Model file for the job. Use its own axes, mm. A direction names the side the tool comes from. Coordinates: 2 decimals unless noted, no trailing zeros. Write each loop counter-clockwise with the first axis right and the second up, starting at its lowest first coordinate (ties: lowest second). Pieces come first, ordered by that corner, then holes. Notation, with made-up numbers: (8.5, 65.5) -> (22.5, 65.5) arc R14 cw to (22.5, 71.5) -> close; hole circle Ø6 at (62.5, -16.5). An arc over 180 degrees is marked (long way). Answer as a JSON object with one key per item and string values. Group by question number.
from build123d import *

# Parameters (mm, degrees)
SKETCH1_W                = 37
SKETCH1_H                = 28
SKETCH1_R                = 1.75
BOSS_EXTRUDE1_DEPTH      = 7.8
BOSS_EXTRUDE2_DEPTH      = 10
BOSS_EXTRUDE2_DEPTH_BACK = 2
SKETCH1_3_W              = 44
SKETCH1_3_H              = 35
SKETCH1_3_W_2            = 37
SKETCH1_3_H_2            = 28
SKETCH1_3_W_3            = 8
SKETCH1_3_H_3            = 3
FILLET1_R                = 9
CUT_EXTRUDE1_DEPTH       = 2.1
HOLE1_D                  = 3.3


with BuildPart() as part:
    # Sketch1 → Boss-Extrude1 (new body)
    with BuildSketch(Plane.XY):
        Polygon((-7.2, 0), (0, 0), (0, 32), (8, 32), (8, 35), (-52, 35), (-52, 32), (-44, 32), (-44, 0), (-36.8, 0), (-36.8, -12), (-7.2, -12), align=None)
        with Locations((-22, 17.5)):
            Rectangle(SKETCH1_W, SKETCH1_H, mode=Mode.SUBTRACT)
        with Locations((-15, -8.4)):
            Circle(SKETCH1_R, mode=Mode.SUBTRACT)
        with Locations((-29, -8.4)):
            Circle(SKETCH1_R, mode=Mode.SUBTRACT)
    extrude(amount=BOSS_EXTRUDE1_DEPTH)

    # Sketch1<3> → Boss-Extrude2 (add, two sides: drawn at the far end of the back side and taken through both)
    # profile 1 of 3: a face of its own
    with BuildSketch(Plane.XY.offset(-BOSS_EXTRUDE2_DEPTH_BACK)):
        with Locations((-22, 17.5)):
            Rectangle(SKETCH1_3_W, SKETCH1_3_H)
        with Locations((-22, 17.5)):
            Rectangle(SKETCH1_3_W_2, SKETCH1_3_H_2, mode=Mode.SUBTRACT)
    # profile 2 of 3: a face of its own
    with BuildSketch(Plane.XY.offset(-BOSS_EXTRUDE2_DEPTH_BACK)):
        with Locations((4, 33.5)):
            Rectangle(SKETCH1_3_W_3, SKETCH1_3_H_3)
    # profile 3 of 3: a face of its own
    with BuildSketch(Plane.XY.offset(-BOSS_EXTRUDE2_DEPTH_BACK)):
        with Locations((-48, 33.5)):
            Rectangle(SKETCH1_3_W_3, SKETCH1_3_H_3)
    extrude(amount=BOSS_EXTRUDE2_DEPTH + BOSS_EXTRUDE2_DEPTH_BACK)

    # Fillet1
    # the kernel refuses this fillet: 9 mm, written as the material it takes off along each edge
    with BuildSketch(Plane(origin=(0, 0, -24.5), x_dir=(-1, 0, 0), z_dir=(0, 0, 1))) as fillet1_piece_1_section:
        with BuildLine():
            CenterArc((FILLET1_R, -FILLET1_R), FILLET1_R, 90, 90)
            Line((0, -FILLET1_R), (0, 0))
            Line((0, 0), (FILLET1_R, 0))
        make_face()
    fillet1_piece_1 = extrude(amount=57, mode=Mode.PRIVATE)
    fillet1_piece_1 = split(fillet1_piece_1, bisect_by=Plane(origin=(-7.2, -0.053721548, -12.25), z_dir=(-1, 0, 0)), keep=Keep.TOP, mode=Mode.PRIVATE)
    fillet1_piece_1 = split(fillet1_piece_1, bisect_by=Plane(origin=(-7.986757567, -0.053721548, 0), z_dir=(0, 0, -1)), keep=Keep.TOP, mode=Mode.PRIVATE)
    add(fillet1_piece_1, mode=Mode.SUBTRACT)
    with BuildSketch(Plane(origin=(0, 0, -24.5), x_dir=(-1, 0, 0), z_dir=(0, 0, 1))) as fillet1_piece_2_section:
        with BuildLine():
            CenterArc((FILLET1_R, -FILLET1_R), FILLET1_R, 90, 90)
            Line((0, -FILLET1_R), (0, 0))
            Line((0, 0), (FILLET1_R, 0))
        make_face()
    fillet1_piece_2 = extrude(amount=57, mode=Mode.PRIVATE)
    fillet1_piece_2 = split(fillet1_piece_2, bisect_by=Plane(origin=(-7.2, 2.082298627, -12.25), z_dir=(1, 0, 0)), keep=Keep.TOP, mode=Mode.PRIVATE)
    fillet1_piece_2 = split(fillet1_piece_2, bisect_by=Plane(origin=(-1.910273674, 2.082298627, 0), z_dir=(0, 0, -1)), keep=Keep.TOP, mode=Mode.PRIVATE)
    add(fillet1_piece_2, mode=Mode.SUBTRACT)
    with BuildSketch(Plane(origin=(0, 0, -24.5), x_dir=(-1, 0, 0), z_dir=(0, 0, 1))) as fillet1_piece_3_section:
        with BuildLine():
            CenterArc((FILLET1_R, -FILLET1_R), FILLET1_R, 90, 90)
            Line((0, -FILLET1_R), (0, 0))
            Line((0, 0), (FILLET1_R, 0))
        make_face()
    fillet1_piece_3 = extrude(amount=57, mode=Mode.PRIVATE)
    fillet1_piece_3 = split(fillet1_piece_3, bisect_by=Plane(origin=(-7.2, 2.082298627, 3.9), z_dir=(1, 0, 0)), keep=Keep.TOP, mode=Mode.PRIVATE)
    fillet1_piece_3 = split(fillet1_piece_3, bisect_by=Plane(origin=(-1.910273674, 2.082298627, 7.8), z_dir=(0, 0, -1)), keep=Keep.TOP, mode=Mode.PRIVATE)
    fillet1_piece_3 = split(fillet1_piece_3, bisect_by=Plane(origin=(-1.910273674, 2.082298627, 0), z_dir=(0, 0, 1)), keep=Keep.TOP, mode=Mode.PRIVATE)
    add(fillet1_piece_3, mode=Mode.SUBTRACT)
    with BuildSketch(Plane(origin=(0, 0, -24.5), x_dir=(-1, 0, 0), z_dir=(0, 0, 1))) as fillet1_piece_4_section:
        with BuildLine():
            CenterArc((FILLET1_R, -FILLET1_R), FILLET1_R, 90, 90)
            Line((0, -FILLET1_R), (0, 0))
            Line((0, 0), (FILLET1_R, 0))
        make_face()
    fillet1_piece_4 = extrude(amount=57, mode=Mode.PRIVATE)
    fillet1_piece_4 = split(fillet1_piece_4, bisect_by=Plane(origin=(-7.2, -0.053721548, 20.15), z_dir=(-1, 0, 0)), keep=Keep.TOP, mode=Mode.PRIVATE)
    fillet1_piece_4 = split(fillet1_piece_4, bisect_by=Plane(origin=(-7.986757567, -0.053721548, 7.8), z_dir=(0, 0, 1)), keep=Keep.TOP, mode=Mode.PRIVATE)
    add(fillet1_piece_4, mode=Mode.SUBTRACT)
    with BuildSketch(Plane(origin=(0, 0, -24.5), x_dir=(-1, 0, 0), z_dir=(0, 0, 1))) as fillet1_piece_5_section:
        with BuildLine():
            CenterArc((FILLET1_R, -FILLET1_R), FILLET1_R, 90, 90)
            Line((0, -FILLET1_R), (0, 0))
            Line((0, 0), (FILLET1_R, 0))
        make_face()
    fillet1_piece_5 = extrude(amount=57, mode=Mode.PRIVATE)
    fillet1_piece_5 = split(fillet1_piece_5, bisect_by=Plane(origin=(-7.2, 2.082298627, 20.15), z_dir=(1, 0, 0)), keep=Keep.TOP, mode=Mode.PRIVATE)
    fillet1_piece_5 = split(fillet1_piece_5, bisect_by=Plane(origin=(-1.910273674, 2.082298627, 7.8), z_dir=(0, 0, 1)), keep=Keep.TOP, mode=Mode.PRIVATE)
    add(fillet1_piece_5, mode=Mode.SUBTRACT)
    with BuildSketch(Plane(origin=(-44, 0, 32.5), x_dir=(1, 0, 0), z_dir=(0, 0, -1))) as fillet1_piece_6_section:
        with BuildLine():
            CenterArc((FILLET1_R, -FILLET1_R), FILLET1_R, 90, 90)
            Line((0, -FILLET1_R), (0, 0))
            Line((0, 0), (FILLET1_R, 0))
        make_face()
    fillet1_piece_6 = extrude(amount=57, mode=Mode.PRIVATE)
    fillet1_piece_6 = split(fillet1_piece_6, bisect_by=Plane(origin=(-36.013242433, -0.053721548, 7.8), z_dir=(0, 0, 1)), keep=Keep.TOP, mode=Mode.PRIVATE)
    fillet1_piece_6 = split(fillet1_piece_6, bisect_by=Plane(origin=(-36.8, -0.053721548, 20.15), z_dir=(1, 0, 0)), keep=Keep.TOP, mode=Mode.PRIVATE)
    add(fillet1_piece_6, mode=Mode.SUBTRACT)
    with BuildSketch(Plane(origin=(-44, 0, 32.5), x_dir=(1, 0, 0), z_dir=(0, 0, -1))) as fillet1_piece_7_section:
        with BuildLine():
            CenterArc((FILLET1_R, -FILLET1_R), FILLET1_R, 90, 90)
            Line((0, -FILLET1_R), (0, 0))
            Line((0, 0), (FILLET1_R, 0))
        make_face()
    fillet1_piece_7 = extrude(amount=57, mode=Mode.PRIVATE)
    fillet1_piece_7 = split(fillet1_piece_7, bisect_by=Plane(origin=(-42.089726326, 2.082298627, 7.8), z_dir=(0, 0, 1)), keep=Keep.TOP, mode=Mode.PRIVATE)
    fillet1_piece_7 = split(fillet1_piece_7, bisect_by=Plane(origin=(-36.8, 2.082298627, 20.15), z_dir=(-1, 0, 0)), keep=Keep.TOP, mode=Mode.PRIVATE)
    add(fillet1_piece_7, mode=Mode.SUBTRACT)
    with BuildSketch(Plane(origin=(-44, 0, 32.5), x_dir=(1, 0, 0), z_dir=(0, 0, -1))) as fillet1_piece_8_section:
        with BuildLine():
            CenterArc((FILLET1_R, -FILLET1_R), FILLET1_R, 90, 90)
            Line((0, -FILLET1_R), (0, 0))
            Line((0, 0), (FILLET1_R, 0))
        make_face()
    fillet1_piece_8 = extrude(amount=57, mode=Mode.PRIVATE)
    fillet1_piece_8 = split(fillet1_piece_8, bisect_by=Plane(origin=(-42.089726326, 2.082298627, 7.8), z_dir=(0, 0, -1)), keep=Keep.TOP, mode=Mode.PRIVATE)
    fillet1_piece_8 = split(fillet1_piece_8, bisect_by=Plane(origin=(-36.8, 2.082298627, 3.9), z_dir=(-1, 0, 0)), keep=Keep.TOP, mode=Mode.PRIVATE)
    fillet1_piece_8 = split(fillet1_piece_8, bisect_by=Plane(origin=(-42.089726326, 2.082298627, 0), z_dir=(0, 0, 1)), keep=Keep.TOP, mode=Mode.PRIVATE)
    add(fillet1_piece_8, mode=Mode.SUBTRACT)
    with BuildSketch(Plane(origin=(-44, 0, 32.5), x_dir=(1, 0, 0), z_dir=(0, 0, -1))) as fillet1_piece_9_section:
        with BuildLine():
            CenterArc((FILLET1_R, -FILLET1_R), FILLET1_R, 90, 90)
            Line((0, -FILLET1_R), (0, 0))
            Line((0, 0), (FILLET1_R, 0))
        make_face()
    fillet1_piece_9 = extrude(amount=57, mode=Mode.PRIVATE)
    fillet1_piece_9 = split(fillet1_piece_9, bisect_by=Plane(origin=(-36.8, -0.053721548, -12.25), z_dir=(1, 0, 0)), keep=Keep.TOP, mode=Mode.PRIVATE)
    fillet1_piece_9 = split(fillet1_piece_9, bisect_by=Plane(origin=(-36.013242433, -0.053721548, 0), z_dir=(0, 0, -1)), keep=Keep.TOP, mode=Mode.PRIVATE)
    add(fillet1_piece_9, mode=Mode.SUBTRACT)
    with BuildSketch(Plane(origin=(-44, 0, 32.5), x_dir=(1, 0, 0), z_dir=(0, 0, -1))) as fillet1_piece_10_section:
        with BuildLine():
            CenterArc((FILLET1_R, -FILLET1_R), FILLET1_R, 90, 90)
            Line((0, -FILLET1_R), (0, 0))
            Line((0, 0), (FILLET1_R, 0))
        make_face()
    fillet1_piece_10 = extrude(amount=57, mode=Mode.PRIVATE)
    fillet1_piece_10 = split(fillet1_piece_10, bisect_by=Plane(origin=(-36.8, 2.082298627, -12.25), z_dir=(-1, 0, 0)), keep=Keep.TOP, mode=Mode.PRIVATE)
    fillet1_piece_10 = split(fillet1_piece_10, bisect_by=Plane(origin=(-42.089726326, 2.082298627, 0), z_dir=(0, 0, -1)), keep=Keep.TOP, mode=Mode.PRIVATE)
    add(fillet1_piece_10, mode=Mode.SUBTRACT)

    # Sketch2 → Cut-Extrude1 (cut)
    with BuildSketch(Plane.XZ.offset(-32)):
        Polygon((-48, 0.449295844), (-44.925, 2.224647922), (-44.925, 5.775352078), (-48, 7.550704156), (-51.075, 5.775352078), (-51.075, 2.224647922), align=None)
        Polygon((0.925, 5.775352078), (0.925, 2.224647922), (4, 0.449295844), (7.075, 2.224647922), (7.075, 5.775352078), (4, 7.550704156), align=None)
    extrude(amount=-CUT_EXTRUDE1_DEPTH, mode=Mode.SUBTRACT)

    # Hole1 (through all)
    with Locations(Plane(origin=(-48, 32, 4), x_dir=(-1, 0, 0), z_dir=(0, -1, 0))):
        with Locations((0, 0), (-52, 0)):
            Hole(HOLE1_D / 2)


solid = part.part
(1) Wall check: probe 1 along X at (y, z) = (34.7, 4); probe 2 along X at (y, z) = (-8.5, 5.25); probe 3 along Z at (x, y) = (-48, 34). Give the ranges that are in metal, low to high.
(2) Cut at A-A on z = 4. Give the number of separate pieces and of enclosed holes in the cut face, plus the area to 3 significant figures.
(3) Pin check, flat tips, straight feed: pin 1 (4 mm diameter, centred on y = -8.5, z = 2.5, fed in from -X); pin 2 (9.5 mm diameter, centred on x = -16, y = -8, fed in from +Z); pin 3 (13.5 mm diameter, centred on x = -24, y = -8, fed in from -Z); pin 4 (4 mm diameter, centred on x = 4, z = 4, fed in from +Y). Stop position of each tip, or through.
(4) Cut at B-B on x = -15. List the corners of the cut face in (y, z).
(5) Cut at C-C on y = 17.5. List the corners of the cut face in (x, z).
(6) Cut at D-D on y = -8.4. List the corners of the cut face in (x, z), plus the area to 3 significant figures.
(7) 3-axis set-ups, long thin cutter, end or side, ignore diameter. For faces 4 (the face through (-50, 32, 1)), 5 (the face through (-7.2, -6, 4)), 6 (the face through (-46.44, 33.04, 6.65)), 7 (the face through (-22, 0, 9)): which of +Z, -Z, +X, -X, +Y, -Y reach the whole face in a straight line?
(8) Pull direction Z, two halves, no side cores. Call faces 1 (the face through (-22, -6, 0)), 2 (the face through (-22, 3.5, 4)), 3 (the face through (-49.65, 34.56, 3.93)): released by +Z, released by -Z, zero draft, split by the parting line, or undercut.
Results found:
{
 "1": {"probe 1": "x = -52 to -49.65, -46.35 to 2.35, 5.65 to 8", "probe 2": "x = -36.8 to -30.75, -27.25 to -16.75, -13.25 to -7.2", "probe 3": "z = -2 to 0.45, 7.55 to 10"},
 "2": {"separate pieces": "3", "enclosed holes": "3", "area": "822 mm²"},
 "3": {"pin 1": "stops at x = -36.8", "pin 2": "stops at z = 7.8", "pin 3": "stops at z = 0", "pin 4": "stops at y = 35"},
 "4": {"outline": "(-12, 0) -> (-10.15, 0) -> (-10.15, 7.8) -> (-12, 7.8) -> close; (-6.65, 0) -> (0, 0) -> (0, -2) -> (3.5, -2) -> (3.5, 10) -> (0, 10) -> (0, 7.8) -> (-6.65, 7.8) -> close; (31.5, -2) -> (35, -2) -> (35, 10) -> (31.5, 10) -> close"},
 "5": {"outline": "(-44, -2) -> (-40.5, -2) -> (-40.5, 10) -> (-44, 10) -> close; (-3.5, -2) -> (0, -2) -> (0, 10) -> (-3.5, 10) -> close"},
 "6": {"outline": "(-36.8, 0) -> (-30.75, 0) -> (-30.75, 7.8) -> (-36.8, 7.8) -> close; (-27.25, 0) -> (-16.75, 0) -> (-16.75, 7.8) -> (-27.25, 7.8) -> close; (-13.25, 0) -> (-7.2, 0) -> (-7.2, 7.8) -> (-13.25, 7.8) -> close", "area": "176 mm²"},
 "7": {"face 4": "+Z, -Z, -X, -Y", "face 5": "+Z, -Z, +X, -Y", "face 6": "-Y", "face 7": "+Z, +X, -X, -Y"},
 "8": {"face 1": "released by -Z", "face 2": "zero draft", "face 3": "undercut"}
}
